Autodesk Inventor part; units mm, degrees
ref_plane "YZ Plane" through (0, 0, 0) normal (1, 0, 0) x (0, 1, 0)
ref_plane "XZ Plane" through (0, 0, 0) normal (0, 1, 0) x (-1, 0, 0)
ref_plane "XY Plane" through (0, 0, 0) normal (0, 0, 1) x (1, 0, 0)
sketch "Sketch1" plane through (0, 0, 0) normal (0, 1, 0) x (-1, 0, 0)
  line L0 (0, 0) -> (0, -61.8744)
  line L1 (0, 0) -> (-3.4036, 0)
  line L2 (0, -61.8744) -> (-3.4036, -61.8744)
  line L3 (-3.4036, 0) -> (-6.5786, -15.5321)
  line L4 (-6.5786, -15.5321) -> (-3.4036, -31.0642)
  line L5 (-3.4036, -31.0642) -> (-6.5786, -46.3423)
  line L6 (-6.5786, -46.3423) -> (-3.4036, -61.8744)
  dimension "d0" = 61.8744
  dimension "d1" = 3.4036
  dimension "d2" = 3.4036
  dimension "d3" = 15.5321
  dimension "d4" = 31.0642
  dimension "d5" = 15.5321
  dimension "d6" = 3.175
  dimension "d7" = 3.175
extrude "Extrusion1" add sketch "Sketch1" along normal blind 7.3025
sketch "Sketch2" plane through (0, 0, 0) normal (0, 0, 1) x (1, 0, 0)
  line L0 (3.4036, 0) -> (0, 0)
  line L1 (0, 7.3025) -> (1.651, 7.3025)
  line L2 (1.651, 7.3025) -> (1.651, 0)
  line L3 (1.651, 0) -> (0, 0)
  line L4 (0, 0) -> (0, 7.3025)
  dimension "d10" = 1.651
sketch "Sketch3" plane through (3.4036, 0, -61.8744) normal (0, 0, -1) x (-1, 0, 0)
  line L0 (0, 0) -> (3.4036, 0)
  line L1 (3.4036, 7.3025) -> (1.7526, 7.3025)
  line L2 (1.7526, 7.3025) -> (1.7526, 0)
  line L3 (1.7526, 0) -> (3.4036, 0)
  line L4 (3.4036, 0) -> (3.4036, 7.3025)
  dimension "d11" = 1.651
extrude "Extrusion2" add sketch "Sketch3" along normal blind 2.5654
extrude "Extrusion3" add sketch "Sketch2" along normal blind 2.5654
properties part number "Short_insert_CPY3"
Model file for the job. Use its own axes, mm. A direction names the side the tool comes from. Round coordinates to 2 decimals unless told otherwise and drop trailing zeros. Order: outer loops, then holes, each group sorted by start corner. A loop starts at its lowest first (then second) coordinate and runs counter-clockwise, first axis right, second up.
(1) 3-axis set-ups, long thin cutter, end or side, ignore diameter. For faces 4 (the face through (3, 4, -61.874)), 5 (the face through (0, 4, -31)), 6 (the face through (1.651, 4, 1)), 7 (the face through (4.97, 3.6, -38.6)): which of +Z, -Z, +X, -X, +Y, -Y reach the whole face in a straight line?
(2) Band-saw the part on D-D (z = -40). List the corners of the cut face in (x, y).
(3) Band-saw the part on A-A (x = 4.5). List the corners of the cut face in (y, z).
(4) Band-saw the part on C-C (z = -32.5). List the corners of the cut face in (x, y).
(5) Pull direction Z, two halves, no side cores. Call faces 1 (the face through (5.013, 3.6, -23.189)), 2 (the face through (1.651, 4, -63)), 3 (the face through (1, 4, -64.44)): released by +Z, released by -Z, zero draft, split by the parting line, or undercut.
(6) Drill centre lines: line 1 (X direction, y = 1.5, z = -53.5); line 2 (X direction, y = 5, z = -22.5). Where is each one in solid material? Low to high.
(7) Pin check, flat tips, straight feed: pin 1 (1.3 mm diameter, centred on y = 2, z = 1, fed in from +X); pin 2 (4 mm diameter, centred on y = 6.5, z = -30.5, fed in from +X); pin 3 (0.9 mm diameter, centred on x = 3, y = 4, fed in from -Z). Stop position of each tip, or through.
(8) Band-saw the part on B-B (y = 6). List the corners of the cut face in (x, z), then the cut area to 3 significant figures.
Verdict:
1. face 4: -Z, +X, +Y, -Y
1. face 5: +Z, -Z, -X, +Y, -Y
1. face 6: +Z, +X, +Y, -Y
1. face 7: +X, +Y, -Y
2. outline: (0, 0) - (5.26, 0) - (5.26, 7.3) - (0, 7.3) - close
3. outline: (0, -56.51) - (7.3, -56.51) - (7.3, -36.34) - (0, -36.34) - close; (0, -25.7) - (7.3, -25.7) - (7.3, -5.36) - (0, -5.36) - close
4. outline: (0, 0) - (3.7, 0) - (3.7, 7.3) - (0, 7.3) - close
5. face 1: undercut
5. face 2: zero draft
5. face 3: released by -Z
6. line 1: x = 0 to 5.12
6. line 2: x = 0 to 5.15
7. pin 1: stops at x = 1.65
7. pin 2: stops at x = 3.93
7. pin 3: stops at z = -61.87
8. outline: (0, -64.44) - (1.65, -64.44) - (1.65, -61.87) - (3.4, -61.87) - (6.58, -46.34) - (3.4, -31.06) - (6.58, -15.53) - (3.4, 0) - (1.65, 0) - (1.65, 2.57) - (0, 2.57) - close
8. area: 317 mm2
